For this review, take the finished solid that the model builds, in its own axes (mm). A direction names the side the tool comes from. Coordinates: 2 decimals unless noted, no trailing zeros. Loops run counter-clockwise (first coordinate to the right, second up) from the corner with the lowest first, then second, coordinate; pieces in that order, holes last.
1. Clearance check with flat-ended pins moving along their axes: P1, Ø8, axis at y = 1, z = -10.5, coming from the +X side; P2, Ø1.5, axis at y = -3.5, z = 5, coming from the +X side; P3, Ø6, axis at x = -5.5, z = -10.5, coming from the +Y side. State where each tip first meets the part, or that it passes through.
2. Take a section at C-C, the plane z = 6.5. State the section outline as (x, y) points (3 decimals), then the cut area to 3 significant figures.
3. Take a section at D-D, the plane z = -12.5. State the section outline as (x, y) points, then the cut area to 3 significant figures.
4. Machinability: for faces 4 (the face through (0, 0, 0)), 5 (the face through (1.36, -6.14, -4.76)), which of the approach directions +Z, -Z, +X, -X, +Y, -Y give a long, thin tool a straight path to every point of the face, cutting with its end or side? Answer none if there is none.
5. To check wall thickness, follow probe 1 along Y at (x, z) = (0, 2) (3 decimals); probe 2 along Z at (x, y) = (-1.5, 5); probe 3 along X at (y, z) = (0.75, 6.25). State the ranges of each line that lie inside material, in increasing order.
6. Mouldability with a two-part tool opening along Y and no side actions: class faces 1 (the face through (0, 0, -15)), 2 (the face through (3.223, 5.055, 5.07)), 3 (the face through (5.77, -1.82, -9.93)) as pulls with the +Y half, pulls with the -Y half, needs draft (parallel to the pull), parting line crosses it, or undercut.
```python
from build123d import *

# Parameters (mm, degrees)
SKETCH1_R           = 11.05
SKETCH1_R_2         = 6.05
BOSS_EXTRUDE1_DEPTH = 10
SKETCH2_R           = 6.05
BOSS_EXTRUDE2_DEPTH = 15
BOSS_EXTRUDE3_START = 5
SKETCH3_R           = 11.05
BOSS_EXTRUDE3_DEPTH = 5
CHAMFER1_SIZE       = 5
SKETCH4_R           = 6.05
SKETCH4_R_2         = 5.995
BOSS_EXTRUDE4_DEPTH = 10


with BuildPart() as part:
    # Sketch1 → Boss-Extrude1 (new body)
    with BuildSketch(Plane.XY):
        Circle(SKETCH1_R)
        Circle(SKETCH1_R_2, mode=Mode.SUBTRACT)
    extrude(amount=BOSS_EXTRUDE1_DEPTH)



with BuildPart() as body_2:
    # Sketch2 → Boss-Extrude2 (new body)
    with BuildSketch(Plane(origin=(0, 0, 0), x_dir=(-1, 0, 0), z_dir=(0, 0, -1))):
        with Locations(Location((0, 0, 0), (0, 0, 180))):
            Circle(SKETCH2_R)
    extrude(amount=BOSS_EXTRUDE2_DEPTH)


with BuildPart() as part_1:
    add(part.part)

    add(body_2.part)  # Boss-Extrude3 merges body 2
    # Sketch3 → Boss-Extrude3 (add)
    with BuildSketch(Plane(origin=(0, 0, 0), x_dir=(-1, 0, 0), z_dir=(0, 0, -1)).offset(BOSS_EXTRUDE3_START)):
        Circle(SKETCH3_R)
    extrude(amount=-BOSS_EXTRUDE3_DEPTH)

    # Chamfer1
    chamfer1_edges = [part_1.edges().sort_by_distance(p)[0] for p in [
        (11.05, 0, -5),
    ]]
    chamfer(chamfer1_edges, length=CHAMFER1_SIZE - 0.0001)  # a hair under: the kernel refuses the full size

    # Sketch4 → Boss-Extrude4 (add)
    with BuildSketch(Plane.XY.offset(10)):
        with Locations(Location((0, 0, 0), (0, 0, 180))):
            Circle(SKETCH4_R)
        Circle(SKETCH4_R_2, mode=Mode.SUBTRACT)
    extrude(amount=-BOSS_EXTRUDE4_DEPTH)


solid = part_1.part
```
Results list:
1. P1: stops at x = 6.05
1. P2: stops at x = 10.7
1. P3: stops at y = 5.51
2. outline: circle Ø22.1 at (0, 0); hole circle Ø11.99 at (0, 0)
2. area: 271 mm2
3. outline: circle Ø12.1 at (0, 0)
3. area: 115 mm2
4. face 4: +Z
4. face 5: -Z
5. probe 1: y = -11.05 to -5.995, 5.995 to 11.05
5. probe 2: z = -15 to 0
5. probe 3: x = -11.02 to -5.95, 5.95 to 11.02
6. face 1: needs draft
6. face 2: undercut
6. face 3: parting line crosses it
